```python
from build123d import *

# Parameters (mm, degrees)
SKETCH1_R           = 7
SKETCH1_R_2         = 6
BOSS_EXTRUDE1_DEPTH = 3.175
SKETCH2_R           = 12.5
SKETCH2_R_2         = 6
BOSS_EXTRUDE2_DEPTH = 1.825
FILLET1_R           = 1


with BuildPart() as part:
    # Sketch1 → Boss-Extrude1 (new body)
    with BuildSketch(Plane(origin=(0, 0, 0), x_dir=(1, 0, 0), z_dir=(0, 1, 0))):
        Circle(SKETCH1_R)
        Circle(SKETCH1_R_2, mode=Mode.SUBTRACT)
    extrude(amount=BOSS_EXTRUDE1_DEPTH)

    # Sketch2 → Boss-Extrude2 (add)
    with BuildSketch(Plane(origin=(0, 3.175, 0), x_dir=(1, 0, 0), z_dir=(0, 1, 0))):
        Circle(SKETCH2_R)
        Circle(SKETCH2_R_2, mode=Mode.SUBTRACT)
    extrude(amount=BOSS_EXTRUDE2_DEPTH)

    # Fillet1
    fillet1_edges = [part.edges().sort_by_distance(p)[0] for p in [
        (-12.5, 5, 0),
    ]]
    fillet(fillet1_edges, radius=FILLET1_R)


solid = part.part
```
Geometry: final body of the model. Coordinates: model frame, mm. Round coordinates to 2 decimals unless told otherwise and drop trailing zeros. Order: outer loops, then holes, each group sorted by start corner. A loop starts at its lowest first (then second) coordinate and runs counter-clockwise, first axis right, second up. Notation, with made-up numbers: (-35.75, 24) - (18.25, 24) arc R26 cw to (18.25, 40) - close; hole circle Ø6 at (-24.75, -26.5). An arc over 180 degrees is marked (long way). Write item = value, one per line. Start each with the question number.
Q1. Cut plane B-B on x = 0. Return the cut outline in (y, z) (3 decimals), and give its area (3 significant figures).
Q2. Cut plane D-D on y = 2.3. Return the cut outline in (x, z).
Q3. Pull-direction query (X, two-part tool) for faces 1 (the flat face through (5.4, 3.175, 5.4)), 2 (the cylindrical face through (-6, 2, 0)), 3 (the cylindrical face through (6.466, 1.565, 2.681)); classes: +X half, -X half, draft (parallel to the pull), parting line (faces both ways), or undercut.
Q4. Ray query, line 1 (X direction, y = 2.25, z = 0); line 2 (Z direction, x = 0, y = 3.8). Return the intervals inside material, ascending. Write a range as from..to.
Q5. Pin query (flat end, axial travel): pin 1 (1.5 mm diameter, centred on y = 2.5, z = 2.5, fed in from +X); pin 2 (3 mm diameter, centred on x = -3.5, y = 2.5, fed in from -Z). Return the tip coordinate at first contact, or that it passes through.
Q6. Cut plane C-C on y = 3.6. Return the cut outline in (x, z), and give its area (3 significant figures).
Q7. Cut plane A-A on z = 0. Return the cut outline in (x, y) (3 decimals).
Outcome:
q1.outline = (0, -7) - (3.175, -7) - (3.175, -12.5) - (4, -12.5) arc R1 ccw to (5, -11.5) - (5, -6) - (0, -6) - close; (0, 6) - (5, 6) - (5, 11.5) arc R1 ccw to (4, 12.5) - (3.175, 12.5) - (3.175, 7) - (0, 7) - close
q1.area = 29.6 mm^2
q2.outline = circle Ø14 at (0, 0); hole circle Ø12 at (0, 0)
q3.face_1 = draft
q3.face_2 = undercut
q3.face_3 = parting line
q4.line_1 = -7..-6, 6..7
q4.line_2 = -12.5..-6, 6..12.5
q5.pin_1 = 12.31
q5.pin_2 = -12.31
q6.outline = circle Ø25 at (0, 0); hole circle Ø12 at (0, 0)
q6.area = 378 mm^2
q7.outline = (-12.5, 3.175) - (-7, 3.175) - (-7, 0) - (-6, 0) - (-6, 5) - (-11.5, 5) arc R1 ccw to (-12.5, 4) - close; (6, 0) - (7, 0) - (7, 3.175) - (12.5, 3.175) - (12.5, 4) arc R1 ccw to (11.5, 5) - (6, 5) - close
